Here's how the part is built. I have some questions about the finished solid (model axes, mm). A direction names the side the tool comes from. Round coordinates to 2 decimals unless told otherwise and drop trailing zeros. Write each loop counter-clockwise with the first axis right and the second up, starting at its lowest first coordinate (ties: lowest second). Pieces come first, ordered by that corner, then holes. Notation, with made-up numbers: (6.25, 9.5) -> (27.25, 9.5) arc R24 cw to (27.25, 19.5) -> close; hole circle Ø7 at (89.5, 29). An arc over 180 degrees is marked (long way). Answer in a Markdown table with one row per item.
from build123d import *

# Parameters (mm, degrees)
F2_SIZE = 0.5
F3_SIZE = 0.5


with BuildPart() as f1:
    # F0 (on Front) → F1 (revolve)
    with BuildSketch(Plane.XZ):
        Polygon((0, 3.5), (0, 0), (0, -6.5), (50, -6.5), (50, 0), (20, 0), (20, 3.5), align=None)
    revolve(axis=Axis((25, 0, -6.5), (-1, 0, 0)))

    # F2
    f2_edges = [f1.edges().sort_by_distance(p)[0] for p in [
        (50, 0, -13),
    ]]
    chamfer(f2_edges, length=F2_SIZE)

    # F3
    f3_edges = [f1.edges().sort_by_distance(p)[0] for p in [
        (20, 0, -16.5),
        (0, 0, -16.5),
    ]]
    chamfer(f3_edges, length=F3_SIZE)


solid = f1.part
1) I need wall thicknesses on line 1 (X direction, y = -6.25, z = -3.75); line 2 (Y direction, x = 46, z = -12); line 3 (Y direction, x = 29.5, z = -5.25). Which ranges of each line are inside material? Lowest first, please. Write a range as [from, to].
Response:
| item | result |
|---|---|
| line 1 | x = [0, 20] |
| line 2 | y = [-3.46, 3.46] |
| line 3 | y = [-6.38, 6.38] |
2) I want a section at B-B, the plane y = 0. List the corners of the cut face in (x, z) for me, and give its area (3 significant figures).
Response:
| item | result |
|---|---|
| outline | (0, -16) -> (0.5, -16.5) -> (19.5, -16.5) -> (20, -16) -> (20, -13) -> (49.5, -13) -> (50, -12.5) -> (50, -0.5) -> (49.5, 0) -> (20, 0) -> (20, 3) -> (19.5, 3.5) -> (0.5, 3.5) -> (0, 3) -> close |
| area | 789 mm^2 |
3) Which directions (+Z, -Z, +X, -X, +Y, -Y) give clear straight access to the entire face, cutting with the end or side of a thin tool? Please do faces 1 (the face through (0, 0, -7)), 2 (the face through (34.54, 1.95, -0.3)).
Response:
| item | result |
|---|---|
| face 1 | +Z, -Z, -X, +Y, -Y |
| face 2 | +X |
4) For pin 1 (8 mm diameter, centred on x = 22, y = 5, fed in from -Z); pin 2 (2 mm diameter, centred on x = 11, y = 5, fed in from -Z); pin 3 (6 mm diameter, centred on x = 41, y = 6.5, fed in from +Z), each with a flat end and sliding along its axis, tell me the tip position at first contact or that it passes through.
Response:
| item | result |
|---|---|
| pin 1 | stops at z = -16.32 |
| pin 2 | stops at z = -15.67 |
| pin 3 | stops at z = -1.02 |
5) I want a section at D-D, the plane x = 8. List the corners of the cut face in (y, z) for me.
Response:
| item | result |
|---|---|
| outline | circle Ø20 at (0, -6.5) |
6) I want a section at C-C, the plane x = 42. List the corners of the cut face in (y, z) for me, and give its area (3 significant figures).
Response:
| item | result |
|---|---|
| outline | circle Ø13 at (0, -6.5) |
| area | 133 mm^2 |
7) I want a section at A-A, the plane z = -6.5. List the corners of the cut face in (x, y) for me, and give its area (3 significant figures).
Response:
| item | result |
|---|---|
| outline | (0, -9.5) -> (0.5, -10) -> (19.5, -10) -> (20, -9.5) -> (20, -6.5) -> (49.5, -6.5) -> (50, -6) -> (50, 6) -> (49.5, 6.5) -> (20, 6.5) -> (20, 9.5) -> (19.5, 10) -> (0.5, 10) -> (0, 9.5) -> close |
| area | 789 mm^2 |
